from build123d import *

# Parameters (mm, degrees)
BOSS_EXTRUDE1_DEPTH     = 0.4
BOSS_EXTRUDE2_START     = -0.1
BOSS_EXTRUDE2_DEPTH     = 0.75
FILLET1_R               = 2
FILLET2_R               = 2
CUT_EXTRUDE1_DEPTH      = 26.275598114
CUT_EXTRUDE1_DEPTH_BACK = 26.275598114
FILLET3_R               = 5
BOSS_EXTRUDE4_DEPTH     = 1.5


with BuildPart() as part:
    # Sketch1 → Boss-Extrude1 (new, symmetric)
    with BuildSketch(Plane.XY):
        Polygon((0, 0), (2, 0), (20.294681103, 11.693172413), (21.054279514, 13.958892298), (0.779302489, 1), (0, 1), align=None)
    extrude(amount=BOSS_EXTRUDE1_DEPTH, both=True)

    # Sketch2 → Boss-Extrude2 (add, symmetric)
    with BuildSketch(Plane.XY.offset(0.4).offset(BOSS_EXTRUDE2_START)):
        Polygon((21.054279514, 13.958892298), (20.717242005, 13.743472434), (19.957643594, 11.47775255), (20.294681103, 11.693172413), align=None)
    extrude(amount=BOSS_EXTRUDE2_DEPTH, both=True)

    # Fillet1
    fillet1_edges = [part.edges().sort_by_distance(p)[0] for p in [
        (0.779302489, 1, 0),
        (2, 0, 0),
    ]]
    fillet(fillet1_edges, radius=FILLET1_R)

    # Fillet2
    # the kernel refuses this fillet: 2 mm, written as the material it adds along each edge
    with BuildSketch(Plane(origin=(21.070401948, 14.796873144, -0.4), x_dir=(-0.9481347144095073, 0.31786878319772466, 0), z_dir=(-0.3178687831977247, -0.9481347144095074, 0))) as fillet2_piece_1_section:
        with BuildLine():
            CenterArc((0.444409721, 2), FILLET2_R, 257.161431859, 12.838568141)
            Line((0, 0.05), (0, 0))
            Line((0, 0), (0.444409721, 0))
        make_face()
    fillet2_piece_1 = extrude(amount=4.611708902, mode=Mode.PRIVATE)
    fillet2_piece_1 = split(fillet2_piece_1, bisect_by=Plane(origin=(21.445983631, 14.209252703, -0.4), z_dir=(0.5385496583097051, -0.8425937725467118, 0)), keep=Keep.TOP, mode=Mode.PRIVATE)
    fillet2_piece_1 = split(fillet2_piece_1, bisect_by=Plane(origin=(22.253808119, 12.945362044, -0.4), z_dir=(-0.538549658309705, 0.8425937725467119, 0)), keep=Keep.TOP, mode=Mode.PRIVATE)
    add(fillet2_piece_1)
    with BuildSketch(Plane(origin=(21.889888122, 17.241225439, 0.4), x_dir=(-0.9481347144095071, 0.3178687831977246, 0), z_dir=(-0.3178687831977247, -0.9481347144095074, 0))) as fillet2_piece_2_section:
        with BuildLine():
            CenterArc((1.475635456, -2), FILLET2_R, 90, 47.545849796)
            Line((0, -0.65), (0, 0))
            Line((0, 0), (1.475635456, 0))
        make_face()
    fillet2_piece_2 = extrude(amount=9.76783758, mode=Mode.PRIVATE)
    fillet2_piece_2 = split(fillet2_piece_2, bisect_by=Plane(origin=(23.136984265, 15.290067496, 0.4), z_dir=(0.5385496583097051, -0.8425937725467118, 0)), keep=Keep.TOP, mode=Mode.PRIVATE)
    fillet2_piece_2 = split(fillet2_piece_2, bisect_by=Plane(origin=(23.944808753, 14.026176837, 0.4), z_dir=(-0.538549658309705, 0.8425937725467119, 0)), keep=Keep.TOP, mode=Mode.PRIVATE)
    add(fillet2_piece_2)

    # Sketch4 → Cut-Extrude1 (cut, two sides: drawn at the far end of the back side and taken through both)
    with BuildSketch(Plane.XY.offset(0.4).offset(-CUT_EXTRUDE1_DEPTH_BACK)):
        Polygon((17.612630282, 13.011216265), (21.976187612, 13.235824871), (21.976187612, 14.520118874), (17.612630282, 14.232504072), align=None)
    extrude(amount=CUT_EXTRUDE1_DEPTH + CUT_EXTRUDE1_DEPTH_BACK, mode=Mode.SUBTRACT)

    # Fillet3
    # the kernel refuses this fillet: 5 mm, written as the material it takes off along each edge
    with BuildSketch(Plane(origin=(19.743162439, 13.120882718, -3.665218242), x_dir=(-0.8425937725466615, -0.5385496583097837, 0), z_dir=(0, 0, 1))) as fillet3_piece_1:
        with BuildLine():
            CenterArc((1.306087297, 5), FILLET3_R, 243.661056807, 26.338943193)
            Line((-0.912314796, 0.519074632), (-0.956682838, 0.429456124))
            ThreePointArc((-0.956682838, 0.429456124), (-0.505609749, 0.172620891), (-0.049452351, -0.086916425))
            Line((-0.049452351, -0.086916425), (0, -0.1))
            Line((0, -0.1), (1.306087297, -0.1))
            Line((1.306087297, -0.1), (1.306087297, 0))
        make_face()
    extrude(amount=7.476378223, mode=Mode.SUBTRACT)

    # Sketch5 → Boss-Extrude4 (add)
    with BuildSketch(Plane.XY.offset(1.05)):
        with BuildLine():
            Line((20.79142067, 13.174840488), (20.294681103, 11.693172413))
            ThreePointArc((20.294681103, 11.693172413), (21.283884924, 12.185636667), (20.79142067, 13.174840488))
        make_face()
    extrude(amount=-BOSS_EXTRUDE4_DEPTH)


solid = part.part
Read the model definition and answer for the solid it produces. Units are mm, in the model's axes. Give positions to 0.01 mm unless a question says otherwise; leave off trailing zeros. Loops run counter-clockwise (first coordinate to the right, second up) from the corner with the lowest first, then second, coordinate; pieces in that order, holes last. Notation, with made-up numbers: (38.25, 67) - (97.25, 67) arc R19 ccw to (97.25, 78) - close; hole circle Ø5 at (-21.75, 87). An arc over 180 degrees is marked (long way). Answer as CSV lines item,"result". Start each with the question number.
1) Find section A-A (z = 0.1). Write down the section's boundary in (x, y), then the cut area to 3 significant figures.
2) Each of these flat-tipped pins is pushed along its axis until it touches: pin 1 Ø1.5 at (x, y) = (4.5, 4.5) entering from -Z; pin 2 Ø4 at (x, y) = (5, 4.5) entering from -Z; pin 3 Ø6 at (x, y) = (5.5, 5) entering from +Z. Where does it stop, or does it pass through?
3) Find section C-C (y = 8). Write down the section's boundary in (x, z), then the cut area to 3 significant figures.
4) Straight lines are drawn through the part: L1, parallel to Z at x = 14.5, y = 9; L2, parallel to X at y = 9.25, z = -0.1; L3, parallel to Y at x = 6, z = -0.25. For each, find the intervals that lie inside material, in ascending order. Write a range as from..to.
5) Find section B-B (x = 13.5). Write down the section's boundary in (y, z).
Findings below:
1,outline,"(0, 0) - (1.42, 0) arc R2 ccw to (2.49, 0.31) - (20.29, 11.69) arc R0.78 ccw to (20.79, 13.17) arc R5 ccw to (18.64, 12.42) - (1.27, 1.31) arc R2 cw to (0.19, 1) - (0, 1) - close"
1,area,"36.1 mm^2"
2,pin 1,"through"
2,pin 2,"z = -0.4"
2,pin 3,"z = 0.4"
3,outline,"(11.73, -0.4) - (14.52, -0.4) - (14.52, 0.4) - (11.73, 0.4) - close"
3,area,"2.23 mm^2"
4,L1,"-0.4..0.4"
4,L2,"13.69..16.47"
4,L3,"2.56..4.34"
5,outline,"(7.35, -0.4) - (9.13, -0.4) - (9.13, 0.4) - (7.35, 0.4) - close"
